from build123d import *

# Parameters (mm, degrees)
ESQUISSE1_R             = 4
BOSS_EXTRU_1_DEPTH      = 20
ESQUISSE2_R             = 4
ESQUISSE2_R_2           = 2.9
BOSS_EXTRU_2_DEPTH      = 17.5
ESQUISSE3_R             = 1.5
ENL_V_MAT_EXTRU_1_DEPTH = 17.5


with BuildPart() as part:
    # Esquisse1 → Boss.-Extru.1 (new body)
    with BuildSketch(Plane.XY):
        with BuildLine():
            Line((-12, 4), (-6, 4))
            Line((-6, 4), (-6, 0))
            ThreePointArc((-6, 0), (0, -6), (6, 0))
            Line((6, 0), (6, 4))
            Line((6, 4), (12, 4))
            Line((12, 4), (12, 8))
            Line((12, 8), (-12, 8))
            Line((-12, 8), (-12, 4))
        make_face()
        Circle(ESQUISSE1_R, mode=Mode.SUBTRACT)
    extrude(amount=-BOSS_EXTRU_1_DEPTH)

    # Esquisse2 → Boss.-Extru.2 (add)
    with BuildSketch(Plane.XY):
        Circle(ESQUISSE2_R)
        Circle(ESQUISSE2_R_2, mode=Mode.SUBTRACT)
    extrude(amount=-BOSS_EXTRU_2_DEPTH)

    # Esquisse3 → Enlèv. mat.-Extru.1 (cut)
    with BuildSketch(Plane.XZ.offset(-4)):
        with Locations(Location((9, -10, 0), (0, 0, 270))):
            Circle(ESQUISSE3_R)
        with Locations(Location((-9, -10, 0), (0, 0, 270))):
            Circle(ESQUISSE3_R)
    extrude(amount=-ENL_V_MAT_EXTRU_1_DEPTH, mode=Mode.SUBTRACT)


solid = part.part
Input: part model. Units: mm. Frame: model coordinates. A direction names the side the tool comes from. Coordinates: 2 decimals unless noted, no trailing zeros. Loops run counter-clockwise (first coordinate to the right, second up) from the corner with the lowest first, then second, coordinate; pieces in that order, holes last.
(1) Section A-A on z = -10. Return the cut outline in (x, y), then the cut area to 3 significant figures.
(2) First-contact query: pin 1 Ø2.5 at (x, z) = (9, -10) entering from -Y; pin 2 Ø4 at (x, y) = (-1, 1) entering from -Z; pin 3 Ø3 at (x, z) = (10, -10.5) entering from -Y; pin 4 Ø3 at (y, z) = (2, -5) entering from -X. Flat tips, straight axial feed; report the tip coordinate or a pass-through.
(3) Section D-D on x = 0. Return the cut outline in (y, z), then the cut area to 4 significant figures.
(4) Material intervals for probe 1 along X at (y, z) = (6.2, -10); probe 2 along Y at (x, z) = (0, -19.15); probe 3 along Y at (x, z) = (0, -3.25), sorted ascending.
(5) Section B-B on x = 9. Return the cut outline in (y, z).
(6) Set-up query: faces 5 (the face through (11, 4, -10)), 6 (the face through (12, 6, -10)), 7 (the face through (-7, 4, -10)). Return all of +Z, -Z, +X, -X, +Y, -Y with unobstructed straight access to the full face (end or side cutting, diameter ignored); none if empty.
(7) Section C-C on y = -2.5. Return the cut outline in (x, z).
(8) Pull-direction query (X, two-part tool) for faces 1 (the face through (-6, 2, -10)), 2 (the face through (3, 1, -17.5)), 3 (the face through (-0.867, -3.905, -18.732)), 4 (the face through (6, 2, -10)); classes: released by +X, released by -X, zero draft, split by the parting line, or undercut.
Data:
1. outline: (-12, 4) - (-10.5, 4) - (-10.5, 8) - (-12, 8) - close; (-7.5, 4) - (-6, 4) - (-6, 0) arc R6 ccw to (6, 0) - (6, 4) - (7.5, 4) - (7.5, 8) - (-7.5, 8) - close; (10.5, 4) - (12, 4) - (12, 8) - (10.5, 8) - close; hole circle Ø5.8 at (0, 0)
1. area: 150 mm2
2. pin 1: passes through
2. pin 2: stops at z = -17.5
2. pin 3: stops at y = 4
2. pin 4: stops at x = -6
3. outline: (-6, -20) - (-4, -20) - (-4, -17.5) - (-2.9, -17.5) - (-2.9, 0) - (-6, 0) - close; (2.9, -17.5) - (4, -17.5) - (4, -20) - (8, -20) - (8, 0) - (2.9, 0) - close
3. area: 158.5 mm2
4. probe 1: x = -12 to -10.5, -7.5 to 7.5, 10.5 to 12
4. probe 2: y = -6 to -4, 4 to 8
4. probe 3: y = -6 to -2.9, 2.9 to 8
5. outline: (4, -20) - (8, -20) - (8, -11.5) - (4, -11.5) - close; (4, -8.5) - (8, -8.5) - (8, 0) - (4, 0) - close
6. face 5: +Z, -Z, +X, -Y
6. face 6: +Z, -Z, +X, +Y, -Y
6. face 7: +Z, -Z, -X, -Y
7. outline: (-5.45, -20) - (-3.12, -20) - (-3.12, -17.5) - (-1.47, -17.5) - (-1.47, 0) - (-5.45, 0) - close; (1.47, -17.5) - (3.12, -17.5) - (3.12, -20) - (5.45, -20) - (5.45, 0) - (1.47, 0) - close
8. face 1: released by -X
8. face 2: undercut
8. face 3: undercut
8. face 4: released by +X
